The listing builds one solid part. Answer for the finished solid, in the listing's coordinates (mm). A direction names the side the tool comes from. Coordinates: 2 decimals unless noted, no trailing zeros. Order: outer loops, then holes, each group sorted by start corner. A loop starts at its lowest first (then second) coordinate and runs counter-clockwise, first axis right, second up. Notation, with made-up numbers: (37, 17.5) -> (92, 17.5) arc R17 cw to (92, 50.5) -> close; hole circle Ø1 at (51, 4). An arc over 180 degrees is marked (long way). Return JSON: item names as keys, results as strings.
from build123d import *

# Parameters (mm, degrees)
SKETCH1_R               = 1.1938
BOSS_EXTRUDE1_DEPTH     = 7.7724
CUT_EXTRUDE1_DEPTH      = 1
CUT_EXTRUDE1_DEPTH_BACK = 8.7724
FILLET1_R               = 2.54


with BuildPart() as part:
    # Sketch1 → Boss-Extrude1 (new body)
    with BuildSketch(Plane.XY):
        with BuildLine():
            Line((-5.065262452, 5.08), (-18.456556559, 5.08))
            ThreePointArc((-18.456556559, 5.08), (-19.426909517, 4.731155792), (-19.953034117, 3.844324324))
            ThreePointArc((-19.953034117, 3.844324324), (-17.981598542, -9.463853015), (-8.128, -18.623587624))
            Line((-8.128, -18.623587624), (-8.128, -17.281160051))
            Line((-8.128, -17.281160051), (2.593084415, -20.153865962))
            ThreePointArc((2.593084415, -20.153865962), (10.900004065, -17.149119843), (17.146958643, -10.903403565))
            Line((17.146958643, -10.903403565), (12.940315476, -3.61728387))
            ThreePointArc((12.940315476, -3.61728387), (12.796393961, -3.475289825), (12.60008731, -3.426922378))
            ThreePointArc((12.60008731, -3.426922378), (9.17217903, -2.398369889), (7.028137334, 0.467212181))
            Line((7.028137334, 0.467212181), (6.053096787, 3.371693793))
            ThreePointArc((6.053096787, 3.371693793), (1.669604011, 7.303273092), (-3.95481445, 5.560217822))
            ThreePointArc((-3.95481445, 5.560217822), (-4.460344292, 5.205196933), (-5.065262452, 5.08))
        make_face()
        with Locations((8.89, -15.24)):
            Circle(SKETCH1_R, mode=Mode.SUBTRACT)
        with BuildLine():
            Line((-3.876453526, 1.038692592), (-3.482013301, 2.510763551))
            ThreePointArc((-3.482013301, 2.510763551), (-2.298514325, 4.447599489), (-0.253578298, 5.432607064))
            Line((-0.253578298, 5.432607064), (-0.201054745, 5.628627633))
            ThreePointArc((-0.201054745, 5.628627633), (-0.082709585, 5.782858048), (0.110030452, 5.808232755))
            Line((0.110030452, 5.808232755), (2.808827211, 5.085092343))
            ThreePointArc((2.808827211, 5.085092343), (2.963057626, 4.966747183), (2.988432333, 4.774007146))
            Line((2.988432333, 4.774007146), (2.93590878, 4.577986577))
            ThreePointArc((2.93590878, 4.577986577), (4.214371541, 2.702476981), (4.270893751, 0.433378367))
            Line((4.270893751, 0.433378367), (3.876453526, -1.038692592))
            ThreePointArc((3.876453526, -1.038692592), (-1.038692592, -3.876453526), (-3.876453526, 1.038692592))
        make_face(mode=Mode.SUBTRACT)
    extrude(amount=-BOSS_EXTRUDE1_DEPTH)

    # Sketch2 → Cut-Extrude1 (cut, two sides)
    with BuildSketch(Plane.XY) as cut_extrude1_sk:
        Polygon((-20.975210343, 86.652654313), (7.028137334, 0.467212181), (12.408372181, -16.091448034), (40.411719858, -102.276890166), (212.782604123, -46.270194811), (151.395673921, 142.659349668), align=None)
    extrude(amount=CUT_EXTRUDE1_DEPTH, mode=Mode.SUBTRACT)
    extrude(cut_extrude1_sk.sketch, amount=-CUT_EXTRUDE1_DEPTH_BACK, mode=Mode.SUBTRACT)

    # Fillet1
    fillet1_edges = [part.edges().sort_by_distance(p)[0] for p in [
        (12.408372181, -16.091448034, -3.8862),
    ]]
    fillet(fillet1_edges, radius=FILLET1_R)


solid = part.part
1. Consider line 1 (X direction, y = 2, z = -5.25); line 2 (Y direction, x = -0.5, z = -6.5); line 3 (X direction, y = -0.25, z = -4.75). Determine where each line is inside the solid, lowest interval first. Write a range as from..to.
Answer block:
{"line 1": "x = -20.22..-3.62, 4.37..6.51", "line 2": "y = -19.33..-3.98, 5.38..7.37", "line 3": "x = -20.32..-4.01, 4.09..7.26"}
2. The part is cut by section B-B on y = -15.24. Give the vertices of the cut face in (x, z).
Answer block:
{"outline": "(-13.44, -7.77) -> (7.7, -7.77) -> (7.7, 0) -> (-13.44, 0) -> close; (10.08, -7.77) -> (11.95, -7.77) -> (11.95, 0) -> (10.08, 0) -> close"}
3. The part is cut by section C-C on x = -1. Give the vertices of the cut face in (y, z), and give its area (3 significant figures).
Answer block:
{"outline": "(-19.19, -7.77) -> (-3.89, -7.77) -> (-3.89, 0) -> (-19.19, 0) -> close; (5.24, -7.77) -> (7.28, -7.77) -> (7.28, 0) -> (5.24, 0) -> close", "area": "135 mm2"}
4. The part is cut by section D-D on x = -10.5. Give the vertices of the cut face in (y, z), and give its area (3 significant figures).
Answer block:
{"outline": "(-17.4, -7.77) -> (5.08, -7.77) -> (5.08, 0) -> (-17.4, 0) -> close", "area": "175 mm2"}
5. The part is cut by section A-A on z = -4. Give the vertices of the cut face in (x, y).
Answer block:
{"outline": "(-19.95, 3.84) arc R20.32 ccw to (-8.13, -18.62) -> (-8.13, -17.28) -> (2.59, -20.15) arc R20.32 ccw to (10.76, -17.24) arc R2.54 ccw to (11.83, -14.3) -> (7.03, 0.47) -> (6.05, 3.37) arc R5.97 ccw to (-3.95, 5.56) arc R1.52 cw to (-5.07, 5.08) -> (-18.46, 5.08) arc R1.52 ccw to start; hole (-3.88, 1.04) arc R4.01 ccw to (3.88, -1.04) -> (4.27, 0.43) arc R4.01 ccw to (2.94, 4.58) -> (2.99, 4.77) arc R0.25 ccw to (2.81, 5.09) -> (0.11, 5.81) arc R0.25 ccw to (-0.2, 5.63) -> (-0.25, 5.43) arc R4.01 ccw to (-3.48, 2.51) -> close; hole circle Ø2.39 at (8.89, -15.24)"}
6. Determine the mould class of faces 1 (the face through (1.44, 5.45, -3.83)), 2 (the face through (6.77, -19.16, -3.83)), 3 (the face through (-4, -6, 0)) for opening direction X: pulls with the +X half, pulls with the -X half, needs draft (parallel to the pull), parting line crosses it, or undercut.
Answer block:
{"face 1": "undercut", "face 2": "pulls with the +X half", "face 3": "needs draft"}
7. Each of these flat-tipped pins is pushed along its axis until it touches: pin 1 Ø1 at (y, z) = (-1.5, -5) entering from -X; pin 2 Ø2 at (x, z) = (3.5, -5) entering from +Y; pin 3 Ø3 at (x, z) = (-13, -6.5) entering from -Y. Where does it stop, or does it pass through?
Answer block:
{"pin 1": "stops at x = -20.3", "pin 2": "stops at y = 7.06", "pin 3": "stops at y = -16.75"}
8. For faces 4 (the face through (-12, 5.08, -4)), 5 (the face through (1.754, 7.284, -3.832)), 6 (the face through (-8.128, -18, -4)), 7 (the face through (-3.682, 1.764, -3.832)), 8 (the face through (6.547, 1.899, -3.832)), determine the directions among +Z, -Z, +X, -X, +Y, -Y from which every point of the face is accessible in a straight line to the end or side of a thin tool.
Answer block:
{"face 4": "+Z, -Z, -X, +Y", "face 5": "+Z, -Z, +Y", "face 6": "+Z, -Z, -Y", "face 7": "+Z, -Z", "face 8": "+Z, -Z, +X, +Y"}
